Design review of the part built by this model. Coordinates are the model's own, in mm. A direction names the side the tool comes from. Round coordinates to 2 decimals unless told otherwise and drop trailing zeros. Loops run counter-clockwise (first coordinate to the right, second up) from the corner with the lowest first, then second, coordinate; pieces in that order, holes last. Notation, with made-up numbers: (59, 31.5) -> (78, 31.5) arc R12 ccw to (78, 47.5) -> close; hole circle Ø4 at (47.5, 86.5). An arc over 180 degrees is marked (long way). Answer as CSV lines item,"result". Start each with the question number.
(1) Machinability: for faces 5 (the face through (-29, 0, 10)), 6 (the face through (-6.084, -2.994, -22.804)), 7 (the face through (-27, 0, 22)), which of the approach directions +Z, -Z, +X, -X, +Y, -Y give a long, thin tool a straight path to every point of the face, cutting with its end or side? Answer none if there is none.
(2) For P1, Ø4.5, axis at y = -21, z = 0, coming from the -X side; P2, Ø4, axis at x = -24, z = -12.5, coming from the -Y side; P3, Ø8, axis at x = -13, y = -10, coming from the +Z side, all flat-tipped, find the tip position at first contact; note any pin that passes through.
(3) Take a section at D-D, the plane y = 18. Write out the cut boundary in (x, z), and give its area (3 significant figures).
(4) Take a section at B-B, the plane y = 0. Write out the cut boundary in (x, z), and give its area (3 significant figures).
(5) Draft analysis for pull direction Y (two halves, no side actions). For faces 1 (the face through (-32.07, 0.26, -19.517)), 2 (the face through (-12, 4, -23)), 3 (the face through (-27, -21, 0)), 4 (the face through (-24.675, 25.865, 10.724)), state which applies: +Y half, -Y half, draft (parallel to the pull), parting line (faces both ways), or undercut.
(6) Take a section at A-A, the plane z = 0. Write out the cut boundary in (x, y).
(7) To check wall thickness, follow line 1 (Z direction, x = -34, y = 0); line 2 (Y direction, x = -19.5, z = 0); line 3 (X direction, y = -19.5, z = -11). State the ranges of each line that lie inside material, in increasing order. Write a range as from..to.
(8) Take a section at C-C, the plane x = -43.5. Write out the cut boundary in (y, z), and give its area (3 significant figures).
Autodesk Fusion 360 part; units mm, degrees
sketch "Sketch1" plane through (0, 0, 0) normal (0, 0, 1) x (1, 0, 0)
  line L0 (0, 0) -> (0, 23)
  line L1 (0, 23) -> (-12, 23)
  line L2 (-12, 23) -> (-12, 28)
  line L3 (-12, 28) -> (-37, 28)
  line L4 (0, 0) -> (-57, 0)
  line L5 (-57, 0) -> (-57, 15)
  line L6 (-57, 15) -> (-37, 15)
  line L7 (-37, 15) -> (-37, 28)
  dimension "d1" = 23
  dimension "d2" = 12
  dimension "d3" = 5
  dimension "d4" = 25
  dimension "d6" = 57
  dimension "d7" = 15
revolve "Revolve1" add sketch "Sketch1" angle 360 about axis through (0, 0, 0) along (-1, 0, 0)
sketch "Sketch2" plane through (-57, 0, 0) normal (-1, 0, 0) x (0, -1, 0)
  circle A0 centre (0, 0) radius 15
  line L0 (0, 0) -> (0, -6)
  line L1 (-4, 4.4721) -> (-4, 10)
  line L2 (4, 4.4721) -> (4, 10)
  line L3 (-4, 10) -> (4, 10)
  arc A1 (-4, 4.4721) -> (4, 4.4721) centre (0, 0) ccw
  dimension "d9" = 12
extrude "Extrude1" cut sketch "Sketch2" against normal through all contours L1 L2 L3 A1
sketch "Sketch3" plane through (-37, 0, 0) normal (-1, 0, 0) x (0, -1, 0)
  circle A0 centre (0, 0) radius 15
  circle A1 centre (0, 0) radius 28
  circle A2 centre (0, 0) radius 21.5 construction
  line L0 (0, 0) -> (0, 21.5) construction
  line L1 (0, 0) -> (21.5, 0) construction
  line L2 (0, 0) -> (0, -21.5) construction
  line L3 (0, 0) -> (-21.5, 0) construction
  circle A3 centre (0, 21.5) radius 2
  circle A4 centre (-21.5, 0) radius 2
  circle A5 centre (0, -21.5) radius 2
  circle A6 centre (21.5, 0) radius 2
  dimension "d18" = 43
  dimension "d19" = 4
  dimension "d21" = 360
extrude "Extrude2" cut sketch "Sketch3" against normal blind 10 contours A3 | A4 | A5 | A6
The answers:
1,face 5,"+X, -X"
1,face 6,"+X"
1,face 7,"-X"
2,P1,"x = -37"
2,P2,"y = -25.96"
2,P3,"z = 27.35"
3,outline,"(-37, -21.45) -> (-12, -21.45) -> (-12, -14.32) -> (0, -14.32) -> (0, 14.32) -> (-12, 14.32) -> (-12, 21.45) -> (-37, 21.45) -> close"
3,area,"1,420 mm²"
4,outline,"(-57, -15) -> (-37, -15) -> (-37, -19.5) -> (-27, -19.5) -> (-27, -23.5) -> (-37, -23.5) -> (-37, -28) -> (-12, -28) -> (-12, -23) -> (0, -23) -> (0, -6) -> (-57, -6) -> close; (-57, 10) -> (0, 10) -> (0, 23) -> (-12, 23) -> (-12, 28) -> (-37, 28) -> (-37, 23.5) -> (-27, 23.5) -> (-27, 19.5) -> (-37, 19.5) -> (-37, 15) -> (-57, 15) -> close"
4,area,"1,560 mm²"
5,face 1,"undercut"
5,face 2,"draft"
5,face 3,"undercut"
5,face 4,"parting line"
6,outline,"(-57, -15) -> (-37, -15) -> (-37, -19.5) -> (-27, -19.5) -> (-27, -23.5) -> (-37, -23.5) -> (-37, -28) -> (-12, -28) -> (-12, -23) -> (0, -23) -> (0, -6) -> (-57, -6) -> close; (-57, 6) -> (0, 6) -> (0, 23) -> (-12, 23) -> (-12, 28) -> (-37, 28) -> (-37, 23.5) -> (-27, 23.5) -> (-27, 19.5) -> (-37, 19.5) -> (-37, 15) -> (-57, 15) -> close"
7,line 1,"-28..-23.5, -19.5..-6, 10..19.5, 23.5..28"
7,line 2,"-28..-6, 6..28"
7,line 3,"-37..0"
8,outline,"circle Ø30 at (0, 0); hole (-4, 4.47) arc R6 ccw (long way) to (4, 4.47) -> (4, 10) -> (-4, 10) -> close"
8,area,"558 mm²"
